Could you check a few things on this model? Use its own coordinates, in mm. Face numbers are marked on the shaded views. A direction names the side the tool comes from. Round coordinates to 2 decimals unless told otherwise and drop trailing zeros. Loops run counter-clockwise (first coordinate to the right, second up) from the corner with the lowest first, then second, coordinate; pieces in that order, holes last. Notation, with made-up numbers: (51, -15.5) -> (89, -15.5) arc R18 ccw to (89, -2.5) -> close; hole circle Ø1 at (33, 14.5). An arc over 180 degrees is marked (long way). Write each question's results on one line, items separated by ' | '. Start each with the question number.
1) Which directions (+Z, -Z, +X, -X, +Y, -Y) give clear straight access to the entire face, cutting with the end or side of a thin tool? Please do the marked faces 1, 2 and 3.
2) Imagine slicing it at D-D, the plane x = -2.2. List the corners of the cut face in (y, z) for me, plus the area to 3 significant figures.
3) Imagine slicing it at B-B, the plane z = 0. List the corners of the cut face in (x, y) for me.
4) If I drill on probe 1 along X at (y, z) = (1.2, 5.05); probe 2 along X at (y, z) = (-0.7, 2.75); probe 3 along X at (y, z) = (-1.6, -4.5), over which ranges is the centre line in solid material (lowest first)?
5) For P1, Ø2, axis at x = 0, z = -5, coming from the -Y side; P2, Ø2, axis at x = 2.5, z = 1, coming from the -Y side; P3, Ø1.5, axis at x = -1.5, z = 1.5, coming from the +Y side; P4, Ø2, axis at x = -2, z = -2, coming from the -Y side, each with a flat end and sliding along its axis, tell me the tip position at first contact or that it passes through.
6) We'd pull the mould along Z, two halves only. Please class the marked faces 4, 5, 6 and 7: pulls with the +Z half, pulls with the -Z half, needs draft (parallel to the pull), parting line crosses it, or undercut.
7) Imagine slicing it at A-A, the plane y = -3.1. List the corners of the cut face in (x, z) for me.
8) Imagine slicing it at C-C, the plane x = 0. List the corners of the cut face in (y, z) for me.
from build123d import *

# Parameters (mm, degrees)
SKETCH_1_W          = 10
SKETCH_1_H          = 12
SKETCH_1_R          = 3.5
EXTRUDE_1_DEPTH     = 1.7
SKETCH_4_W          = 10
SKETCH_4_H          = 12
EXTRUDE_2_DEPTH     = 3.5
CUT_EXTRUDE_START   = 3.5
SKETCH_4_3_W        = 2.4
SKETCH_4_3_H        = 1.9
CUT_EXTRUDE_2_DEPTH = 1.5
SKETCH_5_R          = 0.7
CUT_EXTRUDE_3_DEPTH = 10.382963285
CUT_EXTRUDE_START_2 = -3.7
SKETCH_5_3_R        = 1
CUT_EXTRUDE_4_DEPTH = 1.7
CUT_EXTRUDE_START_3 = -5.2
SKETCH_5_4_R        = 0.3
CUT_EXTRUDE_5_DEPTH = 4


with BuildPart() as part:
    # 草图1 → 凸台-拉伸1 (new body)
    with BuildSketch(Plane(origin=(0, 0, 0), x_dir=(1, 0, 0), z_dir=(0, 1, 0))):
        Rectangle(SKETCH_1_W, SKETCH_1_H)
        with Locations(Location((0, 0, 0), (0, 0, 270))):
            Circle(SKETCH_1_R, mode=Mode.SUBTRACT)
    extrude(amount=EXTRUDE_1_DEPTH)

    # 草图4 → 凸台-拉伸2 (add)
    with BuildSketch(Plane.XZ):
        Rectangle(SKETCH_4_W, SKETCH_4_H)
        with BuildLine():
            Line((3.4, 4.1), (3.4, -1.9))
            ThreePointArc((3.4, -1.9), (2.960660172, -2.960660172), (1.9, -3.4))
            Line((1.9, -3.4), (-1.9, -3.4))
            ThreePointArc((-1.9, -3.4), (-2.960660172, -2.960660172), (-3.4, -1.9))
            Line((-3.4, -1.9), (-3.4, 4.1))
            Line((-3.4, 4.1), (3.4, 4.1))
        make_face(mode=Mode.SUBTRACT)
    extrude(amount=EXTRUDE_2_DEPTH)

    # 草图4<3> → 切除-拉伸2 (cut)
    with BuildSketch(Plane.XZ.offset(CUT_EXTRUDE_START)):
        with Locations((-2.2, 5.05)):
            Rectangle(SKETCH_4_3_W, SKETCH_4_3_H)
        with Locations((2.2, 5.05)):
            Rectangle(SKETCH_4_3_W, SKETCH_4_3_H)
        with BuildLine():
            Line((1.3, -6), (1.3, -3.4))
            Line((1.3, -3.4), (0.830662386, -3.4))
            ThreePointArc((0.830662386, -3.4), (0, -3.5), (-0.830662386, -3.4))
            Line((-0.830662386, -3.4), (-1.3, -3.4))
            Line((-1.3, -3.4), (-1.3, -6))
            Line((-1.3, -6), (1.3, -6))
        make_face()
        with BuildLine():
            ThreePointArc((-0.830662386, -3.4), (0, -3.5), (0.830662386, -3.4))
            Line((0.830662386, -3.4), (-0.830662386, -3.4))
        make_face()
    extrude(amount=-CUT_EXTRUDE_2_DEPTH, mode=Mode.SUBTRACT)

    # 草图5 → 切除-拉伸3 (cut, through all)
    with BuildSketch(Plane(origin=(0, 1.7, 0), x_dir=(1, 0, 0), z_dir=(0, 1, 0))):
        with Locations(Location((0, 4.7, 0), (0, 0, 270))):
            Circle(SKETCH_5_R)
        with Locations(Location((2.2, -5.05, 0), (0, 0, 270))):
            Circle(SKETCH_5_R)
        with Locations(Location((-2.2, -5.05, 0), (0, 0, 270))):
            Circle(SKETCH_5_R)
    extrude(amount=-CUT_EXTRUDE_3_DEPTH, mode=Mode.SUBTRACT)

    # 草图5<3> → 切除-拉伸4 (cut)
    with BuildSketch(Plane(origin=(0, 1.7, 0), x_dir=(1, 0, 0), z_dir=(0, 1, 0)).offset(CUT_EXTRUDE_START_2)):
        with Locations((2.2, -5.05)):
            Circle(SKETCH_5_3_R)
        with Locations((-2.2, -5.05)):
            Circle(SKETCH_5_3_R)
        with Locations(Location((0, 4.7, 0), (0, 0, 90))):
            Circle(SKETCH_5_3_R)
    extrude(amount=CUT_EXTRUDE_4_DEPTH, mode=Mode.SUBTRACT)

    # 草图5<4> → 切除-拉伸5 (cut)
    with BuildSketch(Plane(origin=(0, 1.7, 0), x_dir=(1, 0, 0), z_dir=(0, 1, 0)).offset(CUT_EXTRUDE_START_3)):
        with Locations(Location((3.5, 4.5, 0), (0, 0, 270))):
            Circle(SKETCH_5_4_R)
        with Locations(Location((-3.5, 4.5, 0), (0, 0, 270))):
            Circle(SKETCH_5_4_R)
        with Locations(Location((0, -5.05, 0), (0, 0, 270))):
            Circle(SKETCH_5_4_R)
    extrude(amount=CUT_EXTRUDE_5_DEPTH, mode=Mode.SUBTRACT)


solid = part.part
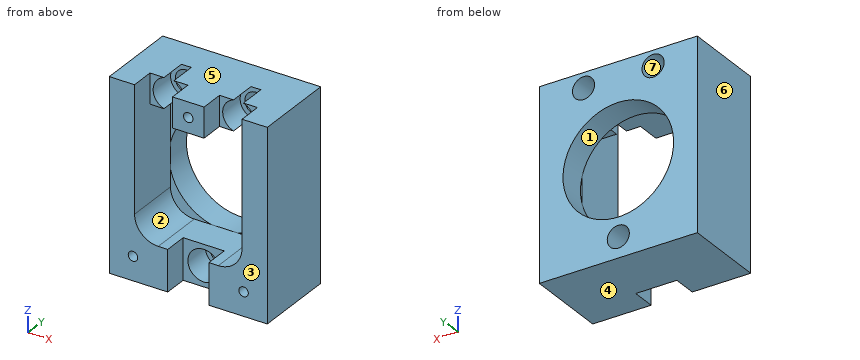
Checked values:
1) face 1: +Y | face 2: -Y | face 3: +Z, -Z, +X, -X, -Y
2) outline: (-3.5, -6) -> (1.7, -6) -> (1.7, -2.72) -> (0, -2.72) -> (0, -3.37) -> (-3.5, -3.37) -> close; (-0.3, 4.1) -> (0, 4.1) -> (0, 2.72) -> (1.7, 2.72) -> (1.7, 4.35) -> (-0.3, 4.35) -> close; (-0.3, 5.75) -> (1.7, 5.75) -> (1.7, 6) -> (-0.3, 6) -> close | area: 18.1 mm^2
3) outline: (-5, -3.5) -> (-3.4, -3.5) -> (-3.4, 0) -> (-3.5, 0) -> (-3.5, 1.7) -> (-5, 1.7) -> close; (3.4, -3.5) -> (5, -3.5) -> (5, 1.7) -> (3.5, 1.7) -> (3.5, 0) -> (3.4, 0) -> close
4) probe 1: -5 to -2.9, -1.5 to 1.5, 2.9 to 5 | probe 2: -5 to -3.4, 3.4 to 5 | probe 3: -5 to -3.8, -3.2 to -0.98, 0.98 to 3.2, 3.8 to 5
5) P1: y = -2 | P2: y = -3.5 | P3: through | P4: y = 0
6) face 4: pulls with the -Z half | face 5: pulls with the +Z half | face 6: needs draft | face 7: undercut
7) outline: (-5, -6) -> (-1.3, -6) -> (-1.3, -3.4) -> (-1.9, -3.4) arc R1.5 cw to (-3.4, -1.9) -> (-3.4, 6) -> (-5, 6) -> close; (-1, 4.1) -> (1, 4.1) -> (1, 6) -> (-1, 6) -> close; (1.3, -6) -> (5, -6) -> (5, 6) -> (3.4, 6) -> (3.4, -1.9) arc R1.5 cw to (1.9, -3.4) -> (1.3, -3.4) -> close; hole circle Ø0.6 at (-3.5, -4.5); hole circle Ø0.6 at (0, 5.05); hole circle Ø0.6 at (3.5, -4.5)
8) outline: (-3.5, 4.1) -> (0, 4.1) -> (0, 3.5) -> (1.7, 3.5) -> (1.7, 6) -> (-3.5, 6) -> (-3.5, 5.35) -> (0.5, 5.35) -> (0.5, 4.75) -> (-3.5, 4.75) -> close; (-2, -6) -> (1.7, -6) -> (1.7, -5.4) -> (-0.3, -5.4) -> (-0.3, -5.7) -> (-2, -5.7) -> close; (-2, -3.7) -> (-0.3, -3.7) -> (-0.3, -4) -> (1.7, -4) -> (1.7, -3.5) -> (0, -3.5) -> (0, -3.4) -> (-2, -3.4) -> close
